```python
from build123d import *

# Parameters (mm, degrees)
SKETCH1_W           = 95.25
SKETCH1_H           = 222.25
BOSS_EXTRUDE1_DEPTH = 6.35
SKETCH2_W           = 17.693613984
SKETCH2_H           = 47.346544424
CUT_EXTRUDE1_DEPTH  = 15.875
CUT_EXTRUDE2_DEPTH  = 6.35
CUT_EXTRUDE3_DEPTH  = 6.35
CUT_EXTRUDE4_DEPTH  = 6.35


with BuildPart() as part:
    # Sketch1 → Boss-Extrude1 (new body)
    with BuildSketch(Plane.XY):
        with Locations((47.625, 111.125)):
            Rectangle(SKETCH1_W, SKETCH1_H)
    extrude(amount=BOSS_EXTRUDE1_DEPTH)

    # Sketch2 → Cut-Extrude1 (cut)
    with BuildSketch(Plane.ZY):
        with Locations((4.668229677, 138.138859748)):
            Rectangle(SKETCH2_W, SKETCH2_H)
    extrude(amount=-CUT_EXTRUDE1_DEPTH, mode=Mode.SUBTRACT)

    # Sketch3 → Cut-Extrude2 (cut)
    with BuildSketch(Plane(origin=(0, 0, 0), x_dir=(-1, 0, 0), z_dir=(0, 0, -1))):
        with BuildLine():
            Line((-51.25, 182.483066433), (-38.55, 182.483066433))
            Line((-38.55, 182.483066433), (-38.55, 118.983066433))
            Line((-38.55, 118.983066433), (-51.25, 118.983066433))
            ThreePointArc((-51.25, 118.983066433), (-55.740128061, 120.842938372), (-57.6, 125.333066433))
            Line((-57.6, 125.333066433), (-57.6, 176.133066433))
            ThreePointArc((-57.6, 176.133066433), (-55.740128061, 180.623194493), (-51.25, 182.483066433))
        make_face()
    extrude(amount=-CUT_EXTRUDE2_DEPTH, mode=Mode.SUBTRACT)

    # Sketch4 → Cut-Extrude3 (cut)
    with BuildSketch(Plane(origin=(0, 0, 0), x_dir=(-1, 0, 0), z_dir=(0, 0, -1))):
        with BuildLine():
            Line((-73.025, 99.100693086), (-22.225, 99.100693086))
            ThreePointArc((-22.225, 99.100693086), (-17.734871939, 97.240821147), (-15.875, 92.750693086))
            Line((-15.875, 92.750693086), (-15.875, 67.350693086))
            ThreePointArc((-15.875, 67.350693086), (-17.734871939, 62.860565025), (-22.225, 61.000693086))
            Line((-22.225, 61.000693086), (-73.025, 61.000693086))
            ThreePointArc((-73.025, 61.000693086), (-77.515128061, 62.860565025), (-79.375, 67.350693086))
            Line((-79.375, 67.350693086), (-79.375, 92.750693086))
            ThreePointArc((-79.375, 92.750693086), (-77.515128061, 97.240821147), (-73.025, 99.100693086))
        make_face()
    extrude(amount=-CUT_EXTRUDE3_DEPTH, mode=Mode.SUBTRACT)

    # Sketch5 → Cut-Extrude4 (cut)
    with BuildSketch(Plane(origin=(0, 0, 0), x_dir=(-1, 0, 0), z_dir=(0, 0, -1))):
        with BuildLine():
            Line((-95.25, 22.225), (-79.248, 22.225))
            Line((-79.248, 22.225), (-79.248, 38.1))
            ThreePointArc((-79.248, 38.1), (-80.17793597, 40.34506403), (-82.423, 41.275))
            Line((-82.423, 41.275), (-95.25, 41.275))
            Line((-95.25, 41.275), (-95.25, 22.225))
        make_face()
        with BuildLine():
            Line((-25.4, 22.225), (-25.4, 38.1))
            ThreePointArc((-25.4, 38.1), (-26.32993597, 40.34506403), (-28.575, 41.275))
            Line((-28.575, 41.275), (-37.973, 41.275))
            ThreePointArc((-37.973, 41.275), (-40.21806403, 40.34506403), (-41.148, 38.1))
            Line((-41.148, 38.1), (-41.148, 22.225))
            Line((-41.148, 22.225), (-25.4, 22.225))
        make_face()
    extrude(amount=-CUT_EXTRUDE4_DEPTH, mode=Mode.SUBTRACT)


solid = part.part
```
Check sheet for the modelled part. Datum: model origin and axes. Units: mm. A direction names the side the tool comes from. Round coordinates to 2 decimals unless told otherwise and drop trailing zeros. Order: outer loops, then holes, each group sorted by start corner. A loop starts at its lowest first (then second) coordinate and runs counter-clockwise, first axis right, second up. Notation, with made-up numbers: (-3.5, 77) -> (30.5, 77) arc R24 cw to (30.5, 107) -> close; hole circle Ø1 at (-7, 77). An arc over 180 degrees is marked (long way). One line per item, written item: value. Start each with the question number.
Q1. Gauge pin test, flat ends, axial feed: pin 1 Ø3 at (y, z) = (133, 3) entering from -X (3 decimals); pin 2 Ø3 at (y, z) = (29, 4.5) entering from +X. Record the tip position at first contact, or that the pin passes through.
Q2. Cross-section at B-B (y = 143). Record the boundary of the cut face in (x, z) (3 decimals), and give its area (3 significant figures).
Q3. Mould release check, pull along Y, two halves, no side actions. Record for faces 4 (the face through (47, 113, 6.35)), 5 (the face through (47, 222.25, 3)), 6 (the face through (55.79, 180.57, 3.13)): pulls with the +Y half, pulls with the -Y half, needs draft (parallel to the pull), parting line crosses it, or undercut.
Q4. Set-up check for faces 1 (the face through (8, 114.466, 3)), 2 (the face through (79.248, 30, 3)), 3 (the face through (33, 22.225, 3)): record each of +Z, -Z, +X, -X, +Y, -Y from which the full face is reachable in a straight line by a thin tool's end or side.
Q5. Thickness scan on line 1 (Y direction, x = 29, z = 0.5) (3 decimals); line 2 (Y direction, x = 52, z = 1.25); line 3 (X direction, y = 27.5, z = 3). Record the ranges inside material, lowest first.
Q6. Cross-section at C-C (z = 3). Give the number of separate pieces and of enclosed holes in the cut face, and give its area (3 significant figures).
Q7. Cross-section at A-A (x = 60). Record the boundary of the cut face in (y, z), and give its area (3 significant figures).
Completed:
1. pin 1: stops at x = 15.875
1. pin 2: stops at x = 79.25
2. outline: (15.875, 0) -> (38.55, 0) -> (38.55, 6.35) -> (15.875, 6.35) -> close; (57.6, 0) -> (95.25, 0) -> (95.25, 6.35) -> (57.6, 6.35) -> close
2. area: 383 mm²
3. face 4: needs draft
3. face 5: pulls with the +Y half
3. face 6: undercut
4. face 1: +Z, -Z, -X
4. face 2: +Z, -Z, +X
4. face 3: +Z, -Z
5. line 1: y = 0 to 22.225, 41.275 to 61.001, 99.101 to 222.25
5. line 2: y = 0 to 61, 99.1 to 119.03, 182.44 to 222.25
5. line 3: x = 0 to 25.4, 41.15 to 79.25
6. separate pieces: 1
6. enclosed holes: 3
6. area: 16,200 mm²
7. outline: (0, 0) -> (61, 0) -> (61, 6.35) -> (0, 6.35) -> close; (99.1, 0) -> (222.25, 0) -> (222.25, 6.35) -> (99.1, 6.35) -> close
7. area: 1,170 mm²
